from build123d import *

# Parameters (mm, degrees)
F0_R     = 1.5
F1_DEPTH = 25
F3_D     = 5
F4_R     = 4
F6_D     = 8
F8_DEPTH = 29.001


with BuildPart() as f1:
    # F0 (on Front) → F1 (new body, symmetric)
    with BuildSketch(Plane.XZ):
        with BuildLine():
            Line((5, 24), (-5, 24))
            Line((-5, 24), (-5, 0))
            ThreePointArc((-5, 0), (0, -5), (5, 0))
            Line((5, 0), (5, 6))
            Line((5, 6), (56, 6))
            Line((56, 6), (56, 16))
            Line((56, 16), (46, 16))
            Line((46, 16), (5, 24))
        make_face()
        with Locations((8, 11)):
            Circle(F0_R, mode=Mode.SUBTRACT)
        with Locations((0, 19)):
            Circle(F0_R, mode=Mode.SUBTRACT)
        with Locations((36, 12)):
            Circle(F0_R, mode=Mode.SUBTRACT)
    extrude(amount=F1_DEPTH, both=True)

    # F3 (through all)
    with Locations(Plane.XZ.offset(25)):
        with Locations((0, 0)):
            Hole(F3_D / 2)

    # F4
    f4_edges = [f1.edges().sort_by_distance(p)[0] for p in [
        (5, 0, 6),
        (5, 0, 24),
        (46, 0, 16),
    ]]
    fillet(f4_edges, radius=F4_R)

    # F6 (through all)
    with Locations(Plane.XY.offset(24)):
        with Locations((50, 0)):
            Hole(F6_D / 2)

    # F7 (on face) → F8 (cut, through all)
    with BuildSketch(Plane.XY.offset(24)):
        Polygon((13, 45), (13, 25), (56, 9), (56, -9), (13, -25), (13, -45), (76, -45), (76, 45), align=None)
    extrude(amount=-F8_DEPTH, mode=Mode.SUBTRACT)


solid = f1.part
The listing builds one solid part. Answer for the finished solid, in the listing's coordinates (mm). A direction names the side the tool comes from. Give positions to 0.01 mm unless a question says otherwise; leave off trailing zeros. Write each loop counter-clockwise with the first axis right and the second up, starting at its lowest first coordinate (ties: lowest second). Pieces come first, ordered by that corner, then holes. Notation, with made-up numbers: (30, 25.25) -> (84, 25.25) arc R21 cw to (84, 41.25) -> close; hole circle Ø9 at (-32.75, 82). An arc over 180 degrees is marked (long way). One line per question, with ' | ' between items. Start each with the question number.
1. Section D-D (y = 7) is taken. Determine the outline of the cut face in (x, z).
2. Section B-B (x = 0) is taken. Determine the outline of the cut face in (y, z).
3. Section C-C (z = 14.25) is taken. Determine the outline of the cut face in (x, y).
4. Section A-A (y = 0) is taken. Determine the outline of the cut face in (x, z), plus the area to 3 significant figures.
5. For faces 1 (the flat face through (54.5, -0.2, 16)), 2 (the flat face through (5, 0, 1)), 3 (the flat face through (-5, 0, 12)), determine the directions among +Z, -Z, +X, -X, +Y, -Y from which every point of the face is accessible in a straight line to the end or side of a thin tool.
6. Given pin 1 Ø12 at (x, z) = (31.5, 20) entering from -Y; pin 2 Ø1 at (x, y) = (31.5, 15) entering from -Z; pin 3 Ø5 at (x, z) = (36, 12) entering from -Y, each flat-ended and moving along its own axis, determine where each tip first touches the part or whether it passes through.
7. Find the intervals of material crossed by probe 1 along X at (y, z) = (6.5, 12.25); probe 2 along Z at (x, y) = (0, 9.5); probe 3 along X at (y, z) = (3, 12), in increasing order.
8. For a pull along Z with two mould halves and no side action, classify faces 4 (the cylindrical face through (0.54, 0.35, -2.44)), 5 (the flat face through (4, -25, 13)), 6 (the cylindrical face through (0, 0, -5)) as pulls with the +Z half, pulls with the -Z half, needs draft (parallel to the pull), parting line crosses it, or undercut.
Response values:
1) outline: (-5, 0) arc R5 ccw to (5, 0) -> (5, 2) arc R4 cw to (9, 6) -> (56, 6) -> (56, 16) -> (46.39, 16) arc R4 cw to (45.62, 16.07) -> (5.38, 23.93) arc R4 ccw to (4.61, 24) -> (-5, 24) -> close; hole circle Ø5 at (0, 0); hole circle Ø3 at (0, 19); hole circle Ø3 at (8, 11); hole circle Ø3 at (36, 12)
2) outline: (-25, -5) -> (25, -5) -> (25, -2.5) -> (-25, -2.5) -> close; (-25, 2.5) -> (25, 2.5) -> (25, 17.5) -> (-25, 17.5) -> close; (-25, 20.5) -> (25, 20.5) -> (25, 24) -> (-25, 24) -> close
3) outline: (-5, -25) -> (13, -25) -> (56, -9) -> (56, 9) -> (13, 25) -> (-5, 25) -> close; hole circle Ø8 at (50, 0)
4) outline: (-5, 0) arc R5 ccw to (5, 0) -> (5, 2) arc R4 cw to (9, 6) -> (46, 6) -> (46, 16.02) arc R4 cw to (45.62, 16.07) -> (5.38, 23.93) arc R4 ccw to (4.61, 24) -> (-5, 24) -> close; (54, 6) -> (56, 6) -> (56, 16) -> (54, 16) -> close; hole circle Ø5 at (0, 0); hole circle Ø3 at (0, 19); hole circle Ø3 at (8, 11); hole circle Ø3 at (36, 12) | area: 836 mm2
5) face 1: +Z, +X, +Y, -Y | face 2: -Z, +X, +Y, -Y | face 3: +Z, -Z, -X, +Y, -Y
6) pin 1: y = -20.35 | pin 2: z = 6 | pin 3: y = -17.37
7) probe 1: -5 to 7.17, 8.83 to 34.52, 37.48 to 56 | probe 2: -5 to -2.5, 2.5 to 17.5, 20.5 to 24 | probe 3: -5 to 6.88, 9.12 to 34.5, 37.5 to 47.35, 52.65 to 56
8) face 4: undercut | face 5: needs draft | face 6: pulls with the -Z half
